Source: CAD feature listing. Evaluate the final solid. Frame: model axes, mm. Give positions to 0.01 mm unless a question says otherwise; leave off trailing zeros. Write each loop counter-clockwise with the first axis right and the second up, starting at its lowest first coordinate (ties: lowest second). Pieces come first, ordered by that corner, then holes. Notation, with made-up numbers: (29, 30) -> (60, 30) arc R31 ccw to (60, 67) -> close; hole circle Ø4 at (45, 70). An arc over 180 degrees is marked (long way). Write item = value, one per line.
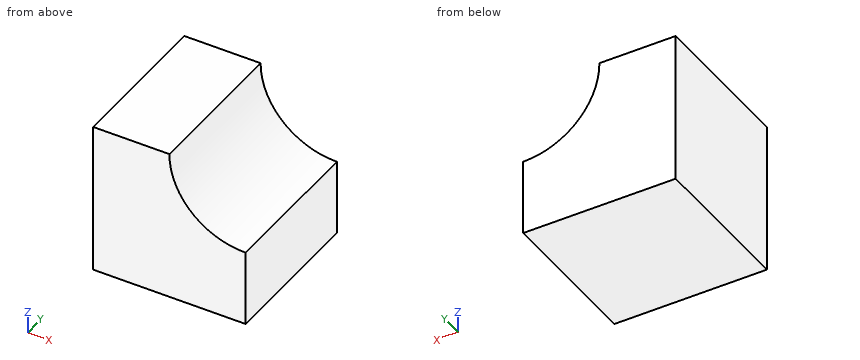
from build123d import *

# Parameters (mm, degrees)
F1_DEPTH = 50.8
F3_DEPTH = 50.8


with BuildPart() as f1:
    # F0 (on Front) → F1 (new body)
    with BuildSketch(Plane.XZ):
        with BuildLine():
            Line((-50.8, 0), (0, 0))
            Line((0, 0), (0, 25.4))
            ThreePointArc((0, 25.4), (-17.970042, 32.829958), (-25.4, 50.8))
            Line((-25.4, 50.8), (-50.8, 50.8))
            Line((-50.8, 50.8), (-50.8, 0))
        make_face()
        with BuildLine():
            ThreePointArc((-25.4, 50.8), (-17.970042, 32.829958), (0, 25.4))
            Line((0, 25.4), (0, 50.8))
            Line((0, 50.8), (-25.4, 50.8))
        make_face()
    extrude(amount=F1_DEPTH)

    # F2 (on face) → F3 (cut)
    with BuildSketch(Plane.XZ.offset(50.8)):
        with BuildLine():
            Line((0, 50.8), (-25.4, 50.8))
            ThreePointArc((-25.4, 50.8), (-17.980258, 32.819742), (0, 25.4))
            Line((0, 25.4), (0, 50.8))
        make_face()
    extrude(amount=-F3_DEPTH, mode=Mode.SUBTRACT)


solid = f1.part
(1) First-contact query: pin 1 (1.5 mm diameter, centred on y = -34, z = 44, fed in from +X); pin 2 (1.5 mm diameter, centred on x = -7, y = -9, fed in from +Z). Flat tips, straight axial feed; report the tip coordinate or a pass-through.
Values follow:
pin_1 = -24.27
pin_2 = 26.59
(2) Section query A-A (y = -25). Return loops of the section in (x, z).
Values follow:
outline = (-50.8, 0) -> (0, 0) -> (0, 25.4) arc R25.33 cw to (-25.4, 50.8) -> (-50.8, 50.8) -> close
(3) Section query B-B (x = -6.5). Return loops of the section in (y, z), plus the area to 3 significant figures.
Values follow:
outline = (-50.8, 0) -> (0, 0) -> (0, 26.23) -> (-50.8, 26.23) -> close
area = 1,330 mm2
(4) Material intervals for line 1 (Z direction, x = -23, y = -26); line 2 (Z direction, x = -3, y = -34); line 3 (X direction, y = -17.5, z = 30), sorted ascending.
Values follow:
line_1 = 0 to 39.97
line_2 = 0 to 25.57
line_3 = -50.8 to -14.62
(5) Section query C-C (z = 40). Return loops of the section in (x, y).
Values follow:
outline = (-50.8, -50.8) -> (-23.01, -50.8) -> (-23.01, 0) -> (-50.8, 0) -> close
